Drawing for the job (mm, zero at the part's lowest x, y, z). Round coordinates to 2 decimals unless told otherwise and drop trailing zeros. Loops run counter-clockwise (first coordinate to the right, second up) from the corner with the lowest first, then second, coordinate; pieces in that order, holes last. Notation, with made-up numbers: (-9, 28.25) - (22, 28.25) arc R14 cw to (22, 38.25) - close; hole circle Ø7 at (8, 37.25). An arc over 180 degrees is marked (long way). Put each result on its own line as item: value.
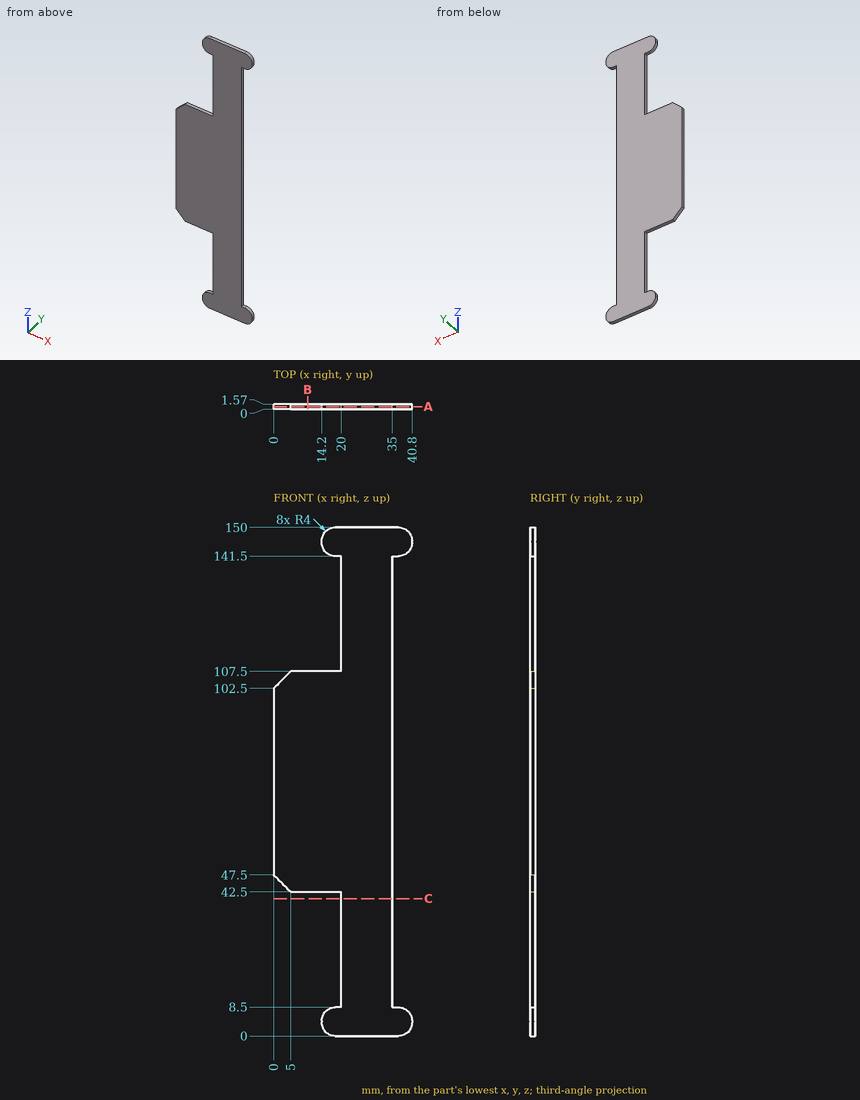
1. Probe line 1 along X through (y, z) = (0.6, 64.5); line 2 along Z through (x, y) = (11, 1.15); line 3 along Z through (x, y) = (39, 0.4). List the from-to ranges inside material, lowest first. Write a range as [from, to].
A:
line 1: x = [0, 35]
line 2: z = [42.5, 107.5]
line 3: z = [0.66, 7.84], [142.16, 149.34]
2. Pin check, flat tips, straight feed: P1, Ø0.8, axis at x = 11.5, y = 1, coming from the +Z side; P2, Ø0.8, axis at y = 0.5, z = 128.5, coming from the -X side. Stop position of each tip, or through.
A:
P1: stops at z = 107.5
P2: stops at x = 20
3. Band-saw the part on C-C (z = 40.5). List the corners of the cut face in (x, y).
A:
outline: (20, 0) - (35, 0) - (35, 1.57) - (20, 1.57) - close
4. Band-saw the part on B-B (x = 10). List the corners of the cut face in (y, z).
A:
outline: (0, 42.5) - (1.57, 42.5) - (1.57, 107.5) - (0, 107.5) - close
5. Band-saw the part on A-A (y = 0.8). List the corners of the cut face in (x, z).
A:
outline: (0, 47.5) - (5, 42.5) - (20, 42.5) - (20, 8.5) - (18.2, 8.5) arc R4 ccw to (14.2, 4.5) - (14.2, 4) arc R4 ccw to (18.2, 0) - (36.8, 0) arc R4 ccw to (40.8, 4) - (40.8, 4.5) arc R4 ccw to (36.8, 8.5) - (35, 8.5) - (35, 141.5) - (36.8, 141.5) arc R4 ccw to (40.8, 145.5) - (40.8, 146) arc R4 ccw to (36.8, 150) - (18.2, 150) arc R4 ccw to (14.2, 146) - (14.2, 145.5) arc R4 ccw to (18.2, 141.5) - (20, 141.5) - (20, 107.5) - (5, 107.5) - (0, 102.5) - close
